Part print with two shaded views. Sizes in mm from the minimum x, y, z corner. Round coordinates to 2 decimals unless told otherwise and drop trailing zeros. Loops run counter-clockwise (first coordinate to the right, second up) from the corner with the lowest first, then second, coordinate; pieces in that order, holes last. Notation, with made-up numbers: M 19.5,70.5 L 64.5,70.5 A30 cw 64.5,100.5 Z; hole C 47.5,2 d11. An arc over 180 degrees is marked long. Use a Markdown table: item, result. Add a question column.
Item 1: Saw through at C-C on y = 17.5. Write the cut outline in (x, z) (1 decimal), then the cut area to 3 significant figures.
Item 2: Saw through at D-D on x = 31. Write the cut outline in (y, z).
Item 3: Pin check, flat tip, straight feed: P1, Ø3, axis at x = 57.5, y = 39, coming from the -Z side. Stop position of the tip, or through.
Item 4: Saw through at A-A on z = 1.5. Write the cut outline in (x, y).
Item 5: Saw through at B-B on x = 61. Write the cut outline in (y, z) (1 decimal).
Item 6: Two-plate mould, pull along Y, no slides. Class the marked faces 1 and 2: +Y half, -Y half, draft (parallel to the pull), parting line (faces both ways), or undercut.
Item 7: Wall check: L1, parallel to Y at x = 82.5, z = 0.65; L2, parallel to X at y = 10.5, z = 1.7; L3, parallel to X at y = 23.5, z = 3.25 (1 decimal). Give the ranges that are in metal, low to high. Write a range as from..to.
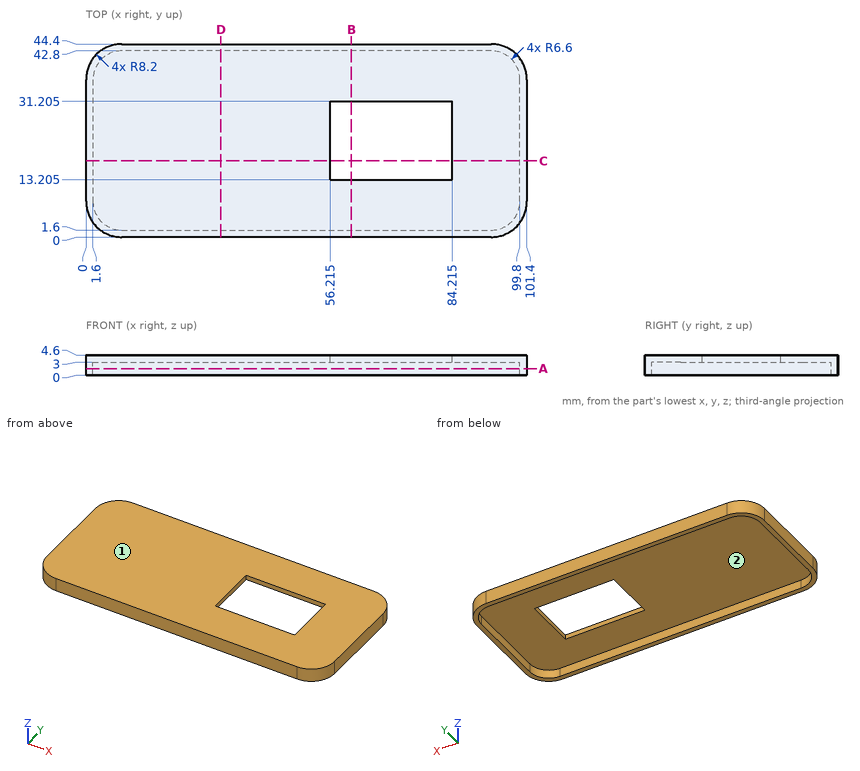
Entries:
| question | item | result |
|---|---|---|
| 1 | outline | M 0,0 L 1.6,0 L 1.6,3 L 56.2,3 L 56.2,4.6 L 0,4.6 Z; M 84.2,3 L 99.8,3 L 99.8,0 L 101.4,0 L 101.4,4.6 L 84.2,4.6 Z |
| 1 | area | 127 mm2 |
| 2 | outline | M 0,0 L 1.6,0 L 1.6,3 L 42.8,3 L 42.8,0 L 44.4,0 L 44.4,4.6 L 0,4.6 Z |
| 3 | P1 | z = 3 |
| 4 | outline | M 0,8.2 A8.2 ccw 8.2,0 L 93.2,0 A8.2 ccw 101.4,8.2 L 101.4,36.2 A8.2 ccw 93.2,44.4 L 8.2,44.4 A8.2 ccw 0,36.2 Z; hole M 1.6,8.2 A6.6 ccw 8.2,1.6 L 93.2,1.6 A6.6 ccw 99.8,8.2 L 99.8,36.2 A6.6 ccw 93.2,42.8 L 8.2,42.8 A6.6 ccw 1.6,36.2 Z |
| 5 | outline | M 0,0 L 1.6,0 L 1.6,3 L 13.2,3 L 13.2,4.6 L 0,4.6 Z; M 31.2,3 L 42.8,3 L 42.8,0 L 44.4,0 L 44.4,4.6 L 31.2,4.6 Z |
| 6 | face 1 | draft |
| 6 | face 2 | undercut |
| 7 | L1 | 0..1.6, 42.8..44.4 |
| 7 | L2 | 0..1.6, 99.8..101.4 |
| 7 | L3 | 0..56.2, 84.2..101.4 |
